Geometry: see drawing. Coordinates: mm, zero at the bounding-box minimum. A direction names the side the tool comes from. Coordinates: 2 decimals unless noted, no trailing zeros. Order: outer loops, then holes, each group sorted by start corner. A loop starts at its lowest first (then second) coordinate and runs counter-clockwise, first axis right, second up.
Item 1: Section B-B on z = 99.5. Return the cut outline in (x, y), then the cut area to 3 significant figures.
Item 2: Ray query, line 1 (Z direction, x = 26, y = 19); line 2 (Y direction, x = 23, z = 100); line 3 (Z direction, x = 43.5, y = 42). Return the intervals inside material, ascending.
Item 3: Section C-C on x = 38.5. Return the cut outline in (y, z).
Item 4: Contact query for flat-ended pins moving along their axis: P1, Ø12, axis at x = 7.5, z = 36.5, coming from the +Y side; P2, Ø10, axis at x = 33.5, z = 83, coming from the +Y side; P3, Ø10, axis at x = 31, z = 15, coming from the +Y side. Output: stop coordinate, or through.
Item 5: Reachability of the marked faces 1, 2, 3, 4 and 5 from +Z, -Z, +X, -X, +Y, -Y: full face, straight path, thin tool, end or side. Return the list, or none.
Item 6: Mould query, pull axis Z, two halves, no side actions, for the marked faces 6, 7 and 8. Classes: released by +Z, released by -Z, zero draft, split by the parting line, or undercut.
Item 7: Section A-A on y = 19. Return the cut outline in (x, z).
Item 8: Section D-D on y = 37. Return the cut outline in (x, z), then the cut area to 3 significant figures.
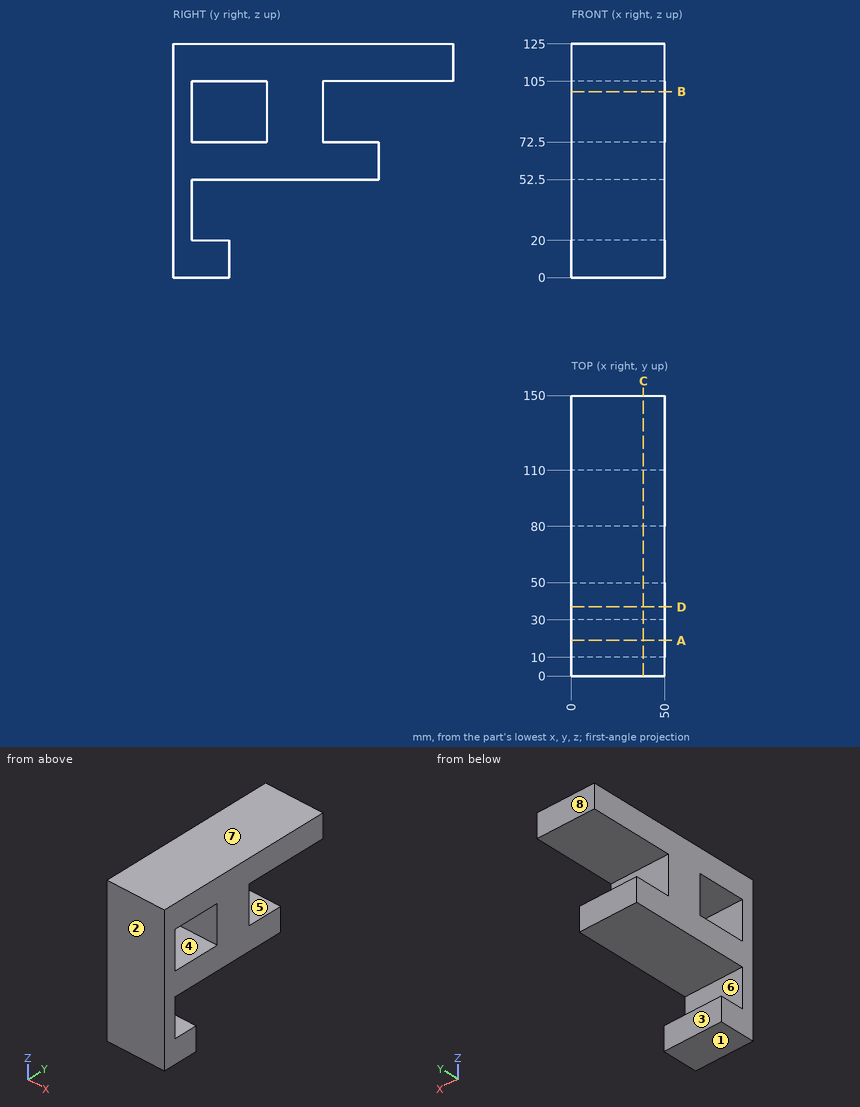
Answer list:
1. outline: (0, 0) - (50, 0) - (50, 10) - (0, 10) - close; (0, 50) - (50, 50) - (50, 80) - (0, 80) - close
1. area: 2,000 mm2
2. line 1: z = 0 to 20, 52.5 to 72.5, 105 to 125
2. line 2: y = 0 to 10, 50 to 80
2. line 3: z = 52.5 to 72.5, 105 to 125
3. outline: (0, 0) - (30, 0) - (30, 20) - (10, 20) - (10, 52.5) - (110, 52.5) - (110, 72.5) - (80, 72.5) - (80, 105) - (150, 105) - (150, 125) - (0, 125) - close; hole (10, 72.5) - (50, 72.5) - (50, 105) - (10, 105) - close
4. P1: stops at y = 10
4. P2: stops at y = 80
4. P3: stops at y = 30
5. face 1: -Z, +X, -X, +Y, -Y
5. face 2: +Z, -Z, +X, -X, -Y
5. face 3: -Z, +X, -X, +Y
5. face 4: +X, -X
5. face 5: +X, -X, +Y
6. face 6: undercut
6. face 7: released by +Z
6. face 8: zero draft
7. outline: (0, 0) - (50, 0) - (50, 20) - (0, 20) - close; (0, 52.5) - (50, 52.5) - (50, 72.5) - (0, 72.5) - close; (0, 105) - (50, 105) - (50, 125) - (0, 125) - close
8. outline: (0, 52.5) - (50, 52.5) - (50, 72.5) - (0, 72.5) - close; (0, 105) - (50, 105) - (50, 125) - (0, 125) - close
8. area: 2,000 mm2
